from build123d import *

# Parameters (mm, degrees)
SKETCH1_R           = 1.7
BOSS_EXTRUDE1_DEPTH = 7
CHAMFER1_SIZE       = 4
CUT_EXTRUDE2_DEPTH  = 23
SKETCH4_R           = 2.7
CUT_EXTRUDE3_DEPTH  = 37
SKETCH5_R           = 1.7
CUT_EXTRUDE4_DEPTH  = 29.5
BOSS_EXTRUDE2_START = -7
SKETCH6_R           = 1.7
BOSS_EXTRUDE2_DEPTH = 7
SKETCH7_R           = 1.7
CUT_EXTRUDE5_DEPTH  = 29.5
CUT_EXTRUDE6_START  = -10
SKETCH9_R           = 1.7
CUT_EXTRUDE6_DEPTH  = 10


with BuildPart() as part:
    # Sketch1 → Boss-Extrude1 (new body)
    # profile 1 of 2: a face of its own
    with BuildSketch(Plane.XY):
        with BuildLine():
            ThreePointArc((151.975863937, 0), (153.975863937, 2), (155.975863937, 0))
            Line((155.975863937, 0), (182.913605213, 0))
            ThreePointArc((182.913605213, 0), (173.710575573, 21.164451961), (151.955140105, 28.867101437))
            ThreePointArc((151.955140105, 28.867101437), (88.828026104, 28.443109388), (26.150636783, 35.976844134))
            ThreePointArc((26.150636783, 35.976844134), (-3.901297619, 28.123718694), (-17.086394787, 0))
            Line((-17.086394787, 0), (10.8, 0))
            ThreePointArc((10.8, 0), (12.5, 1.7), (14.2, 0))
            Line((14.2, 0), (17.5, 0))
            ThreePointArc((17.5, 0), (19.5, 2), (21.5, 0))
            Line((21.5, 0), (24.8, 0))
            ThreePointArc((24.8, 0), (26.5, 1.7), (28.2, 0))
            Line((28.2, 0), (151.975863937, 0))
        make_face()
        with Locations((19.5, 7)):
            Circle(SKETCH1_R, mode=Mode.SUBTRACT)
    # profile 2 of 2: a face of its own
    with BuildSketch(Plane.XY):
        with BuildLine():
            Line((182.913605213, 0), (155.975863937, 0))
            ThreePointArc((155.975863937, 0), (153.975863937, -2), (151.975863937, 0))
            Line((151.975863937, 0), (28.2, 0))
            ThreePointArc((28.2, 0), (26.5, -1.7), (24.8, 0))
            Line((24.8, 0), (21.5, 0))
            ThreePointArc((21.5, 0), (19.5, -2), (17.5, 0))
            Line((17.5, 0), (14.2, 0))
            ThreePointArc((14.2, 0), (12.5, -1.7), (10.8, 0))
            Line((10.8, 0), (-17.086394787, 0))
            ThreePointArc((-17.086394787, 0), (-3.901297619, -28.123718694), (26.150636783, -35.976844134))
            ThreePointArc((26.150636783, -35.976844134), (88.828026104, -28.443109388), (151.955140105, -28.867101437))
            ThreePointArc((151.955140105, -28.867101437), (173.710575573, -21.164451961), (182.913605213, 0))
        make_face()
        with Locations((19.5, -7)):
            Circle(SKETCH1_R, mode=Mode.SUBTRACT)
    extrude(amount=BOSS_EXTRUDE1_DEPTH)

    # Chamfer1
    chamfer1_edges = [part.edges().sort_by_distance(p)[0] for p in [
        (88.828026104, -28.443109388, 7),
        (182.913605213, 0, 7),
        (88.828026104, 28.443109388, 7),
        (-17.086394787, 0, 7),
    ]]
    chamfer(chamfer1_edges, length=CHAMFER1_SIZE)

    # Sketch3 → Cut-Extrude2 (cut)
    with BuildSketch(Plane.XY.offset(7)):
        with BuildLine():
            ThreePointArc((50.964034346, 10.98772537), (38.385340354, 0), (50.964034346, -10.98772537))
            ThreePointArc((50.964034346, -10.98772537), (84.198470815, -7.896690537), (117.575110316, -7.609986123))
            ThreePointArc((117.575110316, -7.609986123), (125.444284006, 0), (117.575110316, 7.609986123))
            ThreePointArc((117.575110316, 7.609986123), (84.198470815, 7.896690537), (50.964034346, 10.98772537))
        make_face()
    extrude(amount=-CUT_EXTRUDE2_DEPTH, mode=Mode.SUBTRACT)

    # Sketch4 → Cut-Extrude3 (cut)
    with BuildSketch(Plane(origin=(0, 0, 0), x_dir=(-1, 0, 0), z_dir=(0, 0, -1))):
        with Locations((-114.313426319, 16.420760727)):
            Circle(SKETCH4_R)
        with Locations((-53.177713255, 20.434899892)):
            Circle(SKETCH4_R)
        with Locations((-114.313426318, -16.420760733)):
            Circle(SKETCH4_R)
        with Locations((-53.177713253, -20.434899892)):
            Circle(SKETCH4_R)
    extrude(amount=-CUT_EXTRUDE3_DEPTH, mode=Mode.SUBTRACT)

    # Sketch5 → Cut-Extrude4 (cut)
    with BuildSketch(Plane(origin=(0, 0, 0), x_dir=(-1, 0, 0), z_dir=(0, 0, -1))):
        with Locations((-19.499999999, -11.235000001)):
            Circle(SKETCH5_R)
        with Locations((-11.555655313, -7.944344687)):
            Circle(SKETCH5_R)
        with Locations((-8.265, -1e-09)):
            Circle(SKETCH5_R)
        with Locations((-11.555655314, 7.944344686)):
            Circle(SKETCH5_R)
        with Locations((-19.500000001, 11.234999999)):
            Circle(SKETCH5_R)
        with Locations((-27.444344687, 7.944344685)):
            Circle(SKETCH5_R)
        with Locations((-30.735, -2e-09)):
            Circle(SKETCH5_R)
        with Locations((-27.444344686, -7.944344688)):
            Circle(SKETCH5_R)
    extrude(amount=-CUT_EXTRUDE4_DEPTH, mode=Mode.SUBTRACT)

    # Sketch6 → Boss-Extrude2 (add)
    with BuildSketch(Plane.XY.offset(7).offset(BOSS_EXTRUDE2_START)):
        with Locations((19.5, 7)):
            Circle(SKETCH6_R)
        with Locations((26.5, 0)):
            Circle(SKETCH6_R)
        with Locations((19.5, -7)):
            Circle(SKETCH6_R)
        with Locations((12.5, 0)):
            Circle(SKETCH6_R)
    extrude(amount=BOSS_EXTRUDE2_DEPTH)

    # Sketch7 → Cut-Extrude5 (cut)
    with BuildSketch(Plane(origin=(0, 0, 0), x_dir=(-1, 0, 0), z_dir=(0, 0, -1))):
        with Locations((-146.03151925, -7.944344686)):
            Circle(SKETCH7_R)
        with Locations((-153.975863936, -11.235)):
            Circle(SKETCH7_R)
        with Locations((-161.920208623, -7.944344687)):
            Circle(SKETCH7_R)
        with Locations((-165.210863937, -1e-09)):
            Circle(SKETCH7_R)
        with Locations((-161.920208624, 7.944344686)):
            Circle(SKETCH7_R)
        with Locations((-153.975863937, 11.235)):
            Circle(SKETCH7_R)
        with Locations((-146.031519251, 7.944344687)):
            Circle(SKETCH7_R)
        with Locations((-142.740863937, 1e-09)):
            Circle(SKETCH7_R)
    extrude(amount=-CUT_EXTRUDE5_DEPTH, mode=Mode.SUBTRACT)

    # Sketch9 → Cut-Extrude6 (cut)
    with BuildSketch(Plane.XY.offset(7).offset(CUT_EXTRUDE6_START)):
        with BuildLine():
            Line((152.275863937, 12.235), (152.275863937, 11.235))
            ThreePointArc((152.275863937, 11.235), (153.975863937, 12.935), (155.675863937, 11.235))
            Line((155.675863937, 11.235), (155.675863937, 12.235))
            ThreePointArc((155.675863937, 12.235), (153.975863937, 13.935), (152.275863937, 12.235))
        make_face()
        with Locations((153.975863937, 11.235)):
            Circle(SKETCH9_R)
        with BuildLine():
            Line((155.675863936, -12.235), (155.675863936, -11.235))
            ThreePointArc((155.675863936, -11.235), (153.975863936, -12.935), (152.275863936, -11.235))
            Line((152.275863939, -11.235), (152.275863939, -12.235))
            ThreePointArc((152.275863939, -12.235), (153.975863937, -13.934999999), (155.675863936, -12.235))
        make_face()
        with Locations((153.975863936, -11.235)):
            Circle(SKETCH9_R)
        with BuildLine():
            ThreePointArc((17.800000001, 11.235), (19.500000001, 12.934999999), (21.200000001, 11.234999999))
            Line((21.199999999, 11.235), (21.199999999, 12.235))
            ThreePointArc((21.199999999, 12.235), (19.499999999, 13.935), (17.799999999, 12.235))
            Line((17.799999999, 12.235), (17.799999999, 11.235))
        make_face()
        with Locations((19.500000001, 11.234999999)):
            Circle(SKETCH9_R)
        with Locations((19.499999999, -11.235000001)):
            Circle(SKETCH9_R)
        with BuildLine():
            ThreePointArc((21.199999999, -11.235000001), (19.499999999, -12.935000001), (17.799999999, -11.235))
            Line((17.800000001, -11.235), (17.800000001, -12.235))
            ThreePointArc((17.800000001, -12.235), (19.499999999, -13.934999999), (21.199999998, -12.235))
            Line((21.199999998, -12.235), (21.199999998, -11.235))
        make_face()
    extrude(amount=CUT_EXTRUDE6_DEPTH, mode=Mode.SUBTRACT)


solid = part.part
Source: CAD feature listing. Evaluate the final solid. Frame: model axes, mm. Give positions to 0.01 mm unless a question says otherwise; leave off trailing zeros. Return JSON: item names as keys, results as strings. Group by question number.
1) Draft query along Y for faces 1 (the face through (163.27, 6.91, 3.45)), 2 (the face through (9.934, -7.434, 3.451)), 3 (the face through (82, 9, 0)), 4 (the face through (87.945, -28.494, 1.479)). Return one class per face: released by +Y, released by -Y, zero draft, split by the parting line, or undercut.
2) Ray query, L1, parallel to Y at x = 51, z = 2; L2, parallel to X at y = 11.5, z = 3.5; L3, parallel to X at y = -13, z = 5.25. Return the intervals inside material, ascending.
3) First-contact query: pin 1 Ø4 at (y, z) = (17, 0.5) entering from -X; pin 2 Ø1.1 at (y, z) = (-11.5, 3) entering from -X; pin 3 Ø1.1 at (y, z) = (-11.5, 4.5) entering from +X. Flat tips, straight axial feed; report the tip coordinate or a pass-through.
Data:
{
 "1": {"face 1": "undercut", "face 2": "undercut", "face 3": "zero draft", "face 4": "released by -Y"},
 "2": {"L1": "y = -32.03 to -22.03, -18.84 to -10.98, 10.98 to 18.84, 22.03 to 32.03", "L2": "x = -14.7 to 17.8, 21.2 to 152.28, 155.68 to 179.98", "L3": "x = -12.28 to 17.98, 21.02 to 152.46, 155.49 to 177.28"},
 "3": {"pin 1": "stops at x = -13.87", "pin 2": "stops at x = -15.41", "pin 3": "stops at x = 179.54"}
}
